```python
from build123d import *

# Parameters (mm, degrees)
F0_R     = 10
F1_DEPTH = 10
F2_W     = 32
F2_H     = 10
F3_DEPTH = 10
F4_R     = 1.625
F5_DEPTH = 25
F6_R     = 3
F7_DEPTH = 3
F8_W     = 5
F8_H     = 20
F9_DEPTH = 5


with BuildPart() as f1:
    # F0 (on Top) → F1 (new body)
    with BuildSketch(Plane.XY):
        with BuildLine():
            Line((-25, -16), (0, -16))
            ThreePointArc((0, -16), (16, 0), (0, 16))
            Line((0, 16), (-25, 16))
            Line((-25, 16), (-25, -16))
        make_face()
        Circle(F0_R, mode=Mode.SUBTRACT)
    extrude(amount=F1_DEPTH)

    # F2 (on face) → F3 (join)
    with BuildSketch(Plane(origin=(-25, 0, 0), x_dir=(0, -1, 0), z_dir=(-1, 0, 0))):
        with Locations((0, 15)):
            Rectangle(F2_W, F2_H)
    extrude(amount=-F3_DEPTH)

    # F4 (on face) → F5 (cut)
    with BuildSketch(Plane.YZ.offset(-15)):
        with Locations((0, 15)):
            Circle(F4_R)
    extrude(amount=-F5_DEPTH, mode=Mode.SUBTRACT)

    # F6 (on face) → F7 (cut)
    with BuildSketch(Plane.YZ.offset(-15)):
        with Locations((0, 15)):
            Circle(F6_R)
    extrude(amount=-F7_DEPTH, mode=Mode.SUBTRACT)

    # F8 (on face) → F9 (join)
    with BuildSketch(Plane(origin=(-25, 0, 0), x_dir=(0, -1, 0), z_dir=(-1, 0, 0))):
        with Locations((13.5, 10)):
            Rectangle(F8_W, F8_H)
    extrude(amount=F9_DEPTH)


solid = f1.part
```
Here's how the part is built. I have some questions about the finished solid (model axes, mm). A direction names the side the tool comes from. Give positions to 0.01 mm unless a question says otherwise; leave off trailing zeros. Loops run counter-clockwise (first coordinate to the right, second up) from the corner with the lowest first, then second, coordinate; pieces in that order, holes last. Notation, with made-up numbers: M -25,70 L 33,70 A24 ccw 33,100 Z; hole C 26.25,-23 d10. An arc over 180 degrees is marked long. Put each result on its own line as item: value. Start each with the question number.
(1) I want a section at B-B on z = 15. Please give me the cut outline in (x, y) (3 decimals).
(2) I want a section at C-C on x = 7. Please give me the cut outline in (y, z).
(3) For faces 4 (the cylindrical face through (-16.48, -0.65, 12.07)), 5 (the flat face through (-10, -3, 10)), 6 (the flat face through (-18, -16, 8)), 7 (the flat face through (-25, 3, 10)), which set-ups out of +Z, -Z, +X, -X, +Y, -Y let a thin tool reach every point of the face, with its end or its side?
(4) If we mould it in two halves opening along Z, with no side actions, what happens to faces 1 (the flat face through (-12, 0, 0)), 2 (the flat face through (-18, 1.3, 13.7)), 3 (the flat face through (-15, 0.2, 11.7))? For each: +Z half, -Z half, draft (parallel to the pull), parting line (faces both ways), or undercut.
(5) I want a section at A-A on y = 0. Please give me the cut outline in (x, z) (3 decimals), then the cut area to 3 significant figures.
(6) I need wall thicknesses on line 1 along Z through (x, y) = (-20, 0) (3 decimals); line 2 along Z through (x, y) = (-16, 0); line 3 along X through (y, z) = (9, 18). Which ranges of each line are inside material? Lowest first, please. Write a range as [from, to].
(7) Will these pins go through, and if not, where does the flat tip stop? pin 1 Ø12 at (x, z) = (-10.5, 16) entering from -Y; pin 2 Ø4 at (x, z) = (-27.5, 14) entering from +Y; pin 3 Ø6.5 at (y, z) = (-1.5, 16) entering from +X; pin 4 Ø6 at (y, z) = (-4, 4) entering from -X.
(8) I want a section at D-D on z = 5.5. Please give me the cut outline in (x, y).
Answer block:
1. outline: M -30,-16 L -15,-16 L -15,-3 L -18,-3 L -18,-1.625 L -25,-1.625 L -25,-11 L -30,-11 Z; M -25,1.625 L -18,1.625 L -18,3 L -15,3 L -15,16 L -25,16 Z
2. outline: M -14.39,0 L -7.14,0 L -7.14,10 L -14.39,10 Z; M 7.14,0 L 14.39,0 L 14.39,10 L 7.14,10 Z
3. face 4: +X
3. face 5: +Z, +X, +Y, -Y
3. face 6: +Z, -Z, +X, -X, -Y
3. face 7: +Z, -Z, -X, +Y
4. face 1: -Z half
4. face 2: undercut
4. face 3: draft
5. outline: M -25,0 L -10,0 L -10,10 L -15,10 L -15,12 L -18,12 L -18,13.375 L -25,13.375 Z; M -25,16.625 L -18,16.625 L -18,18 L -15,18 L -15,20 L -25,20 Z; M 10,0 L 16,0 L 16,10 L 10,10 Z
5. area: 269 mm^2
6. line 1: [0, 13.375], [16.625, 20]
6. line 2: [0, 12], [18, 20]
6. line 3: [-25, -15]
7. pin 1: y = -16
7. pin 2: y = -11
7. pin 3: x = -15
7. pin 4: x = -25
8. outline: M -30,-16 L 0,-16 A16 ccw 0,16 L -25,16 L -25,-11 L -30,-11 Z; hole C 0,0 d20
